```python
from build123d import *

# Parameters (mm, degrees)
F0_R     = 1
F1_DEPTH = 5
F2_R     = 1.5
F3_DEPTH = 10
F4_F1_R  = 1
F4_F2_R  = 1


with BuildPart() as f1:
    # F0 (on Top) → F1 (new body)
    with BuildSketch(Plane.XY):
        with BuildLine():
            Line((13.1224989992, 2.5), (3.1224989992, 2.5))
            ThreePointArc((3.1224989992, 2.5), (-4, 0), (3.1224989992, -2.5))
            Line((3.1224989992, -2.5), (13.1224989992, -2.5))
            Line((13.1224989992, -2.5), (13.1224989992, 2.5))
        make_face()
        Circle(F0_R, mode=Mode.SUBTRACT)
    extrude(amount=F1_DEPTH)

    # F2 (on face) → F3 (cut)
    with BuildSketch(Plane.YZ.offset(13.1224989992)):
        with Locations((0, 2.5)):
            Circle(F2_R)
    extrude(amount=-F3_DEPTH, mode=Mode.SUBTRACT)

    # F4: fillet of radius 1 on 4 edges, made by hand

    # F4_f1
    f4_f1_edges = [f1.edges().sort_by_distance(p)[0] for p in [
        (3.1224989992, 2.5, 2.5),
        (3.1224989992, -2.5, 2.5),
    ]]
    fillet(f4_f1_edges, radius=F4_F1_R)

    # F4_f2
    f4_f2_edges = [f1.edges().sort_by_distance(p)[0] for p in [
        (8.3466066067, -2.5, 5),
        (8.3466066067, -2.5, 0),
        (3.1834158797, -2.5780455543, 0),
        (3.1834158797, -2.5780455543, 5),
    ]]
    fillet(f4_f2_edges, radius=F4_F2_R)


solid = f1.part
```
For this review, take the finished solid that the model builds, in its own axes (mm). A direction names the side the tool comes from. Round coordinates to 2 decimals unless told otherwise and drop trailing zeros. Write each loop counter-clockwise with the first axis right and the second up, starting at its lowest first coordinate (ties: lowest second). Pieces come first, ordered by that corner, then holes. Notation, with made-up numbers: M 30.5,2.5 L 56.5,2.5 A19 ccw 56.5,39.5 Z; hole C -18,11.5 d2. An arc over 180 degrees is marked long. One line per item, written item: value. Start each with the question number.
(1) Wall thickness on line 1 (Z direction, x = 12, y = 0); line 2 (Y direction, x = 0, z = 3.1); line 3 (Y direction, x = 10.5, z = 1.6): over which ranges is each line inside the solid? List them lowest first.
(2) We need section C-C (x = 6). Give the boundary of the cut face in (y, z).
(3) Machinability: for faces 1 (the flat face through (8, 2.5, 2)), 2 (the cylindrical face through (8.28, 2.199, 4.715)), 3 (the cylindrical face through (8.413, -2.199, 0.285)), 4 (the cylindrical face through (8.28, 2.199, 0.285)), 5 (the cylindrical face through (8, 0, 1)), which of the approach directions +Z, -Z, +X, -X, +Y, -Y give a long, thin tool a straight path to every point of the face, cutting with its end or side? Answer none if there is none.
(4) Insertion check: pin 1 (1.5 mm diameter, centred on x = 10.5, z = 2, fed in from +Y); pin 2 (1.8 mm diameter, centred on y = 0, z = 2.5, fed in from +X); pin 3 (1.5 mm diameter, centred on x = 10.5, z = 2.5, fed in from -Y). Each pin has a flat end and moves straight along its axis. Give the tip position at first contact, or say it passes through.
(5) We need section B-B (z = 2.5). Give the boundary of the cut face in (x, y), and give its area (3 significant figures).
(6) The part is to be moulded in two halves that separate along X. For faces 6 (the cylindrical face through (-4, 0, 2)), 7 (the cylindrical face through (0, -1, 2)), 8 (the flat face through (3.122, 0, 3)), say which applies: released by +X, released by -X, zero draft, split by the parting line, or undercut.
(7) We need section D-D (z = 0.65). Give the boundary of the cut face in (x, y).
(8) We need section A-A (y = 0). Give the boundary of the cut face in (x, z), and give its area (3 significant figures).
Result:
1. line 1: 0 to 1, 4 to 5
1. line 2: -4 to -1, 1 to 4
1. line 3: -2.5 to -1.2, 1.2 to 2.5
2. outline: M -2.5,1 A1 ccw -1.5,0 L 1.5,0 A1 ccw 2.5,1 L 2.5,4 A1 ccw 1.5,5 L -1.5,5 A1 ccw -2.5,4 Z; hole C 0,2.5 d3
3. face 1: +Z, -Z, +X, +Y
3. face 2: +Z, +X, +Y
3. face 3: -Z, +X, -Y
3. face 4: -Z, +X, +Y
3. face 5: +X
4. pin 1: y = 2.5
4. pin 2: x = 3.12
4. pin 3: y = -2.5
5. outline: M 2.86,-2.8 A1 cw 3.57,-2.5 L 13.12,-2.5 L 13.12,-1.5 L 3.12,-1.5 L 3.12,1.5 L 13.12,1.5 L 13.12,2.5 L 3.57,2.5 A1 cw 2.86,2.8 A4 ccw long Z; hole C 0,0 d2
5. area: 64.2 mm²
6. face 6: split by the parting line
6. face 7: undercut
6. face 8: released by +X
7. outline: M 2.81,-2.76 A1.06 cw 3.57,-2.44 L 13.12,-2.44 L 13.12,2.44 L 3.57,2.44 A1.06 cw 2.81,2.76 A3.94 ccw long Z; hole C 0,0 d2
8. outline: M -4,1 A1 ccw -3,0 L -1,0 L -1,5 L -3,5 A1 ccw -4,4 Z; M 1,0 L 13.12,0 L 13.12,1 L 3.12,1 L 3.12,4 L 13.12,4 L 13.12,5 L 1,5 Z
8. area: 45.2 mm²
